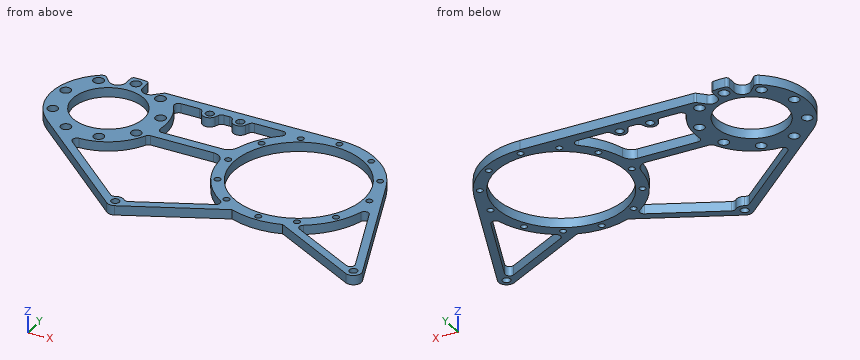
```python
from build123d import *
from build123d.topology import SkipClean

# Parameters (mm, degrees)
SKETCH2_R               = 28.575
SKETCH2_R_2             = 3.2639
SKETCH2_R_3             = 52.3875
BOSS_EXTRUDE1_DEPTH     = 7.62
CUT_EXTRUDE1_DEPTH      = 369.573342704
CUT_EXTRUDE1_DEPTH_BACK = 369.573342704
SKETCH3_R               = 4.15
SKETCH3_R_2             = 2.5
CUT_EXTRUDE2_DEPTH      = 369.573342704
CUT_EXTRUDE2_DEPTH_BACK = 369.573342704
BOSS_EXTRUDE2_DEPTH     = 7.62
CUT_EXTRUDE3_DEPTH      = 369.573342704
CUT_EXTRUDE3_DEPTH_BACK = 369.573342704
SKETCH12_R              = 3.2639


with BuildPart() as part:
    # Sketch2 → Boss-Extrude1 (new body)
    with BuildSketch(Plane.XY):
        with BuildLine():
            Line((-308.866129262, 91.710399516), (-215.926365234, 14.107506231))
            ThreePointArc((-215.926365234, 14.107506231), (-212.572921228, 12.657721799), (-208.970475069, 13.265869211))
            Line((-208.970475069, 13.265869211), (-134.814952137, 49.535152614))
            ThreePointArc((-134.814952137, 49.535152614), (-114.3, 46.0375), (-93.785047863, 49.535152614))
            Line((-93.785047863, 49.535152614), (-21.949808906, 13.301039962))
            ThreePointArc((-21.949808906, 13.301039962), (-14.699565425, 14.303090245), (-13.070560605, 21.438668609))
            Line((-13.070560605, 21.438668609), (-56.805390428, 130.917967399))
            ThreePointArc((-56.805390428, 130.917967399), (-80.468257666, 159.801430712), (-116.436314755, 169.825631839))
            Line((-116.436314755, 169.825631839), (-254.491729173, 165.059137987))
            ThreePointArc((-254.491729173, 165.059137987), (-255.416448823, 164.850182772), (-256.200136715, 164.316701751))
            Line((-256.200136715, 164.316701751), (-261.465020333, 159.051818133))
            ThreePointArc((-261.465020333, 159.051818133), (-268.548656721, 157.642795249), (-272.56121441, 163.648012211))
            Line((-272.56121441, 163.648012211), (-272.56121441, 170.220745001))
            ThreePointArc((-272.56121441, 170.220745001), (-273.218379704, 171.925600851), (-274.84982344, 172.748273949))
            ThreePointArc((-274.84982344, 172.748273949), (-279.4, 172.974), (-283.95017656, 172.748273949))
            ThreePointArc((-283.95017656, 172.748273949), (-285.581620296, 171.925600851), (-286.23878559, 170.220745001))
            Line((-286.23878559, 170.220745001), (-286.23878559, 163.648012211))
            ThreePointArc((-286.23878559, 163.648012211), (-290.251343279, 157.642795249), (-297.334979667, 159.051818133))
            Line((-297.334979667, 159.051818133), (-302.027964646, 163.744803112))
            ThreePointArc((-302.027964646, 163.744803112), (-304.229986022, 164.757469568), (-306.560860086, 164.09307692))
            ThreePointArc((-306.560860086, 164.09307692), (-325.350701602, 128.463454238), (-308.866129262, 91.710399516))
        make_face()
        with Locations(Location((-279.4, 127, 0), (0, 0, 180))):
            Circle(SKETCH2_R, mode=Mode.SUBTRACT)
        with Locations(Location((-19.05, 19.05, 0), (0, 0, 180))):
            Circle(SKETCH2_R_2, mode=Mode.SUBTRACT)
        with Locations(Location((-211.799479175, 19.05, 0), (0, 0, 180))):
            Circle(SKETCH2_R_2, mode=Mode.SUBTRACT)
        with Locations(Location((-114.3, 107.95, 0), (0, 0, 180))):
            Circle(SKETCH2_R_3, mode=Mode.SUBTRACT)
    extrude(amount=BOSS_EXTRUDE1_DEPTH)

    # Sketch3 → Cut-Extrude1 (cut, two sides: drawn at the far end of the back side and taken through both)
    with BuildSketch(Plane.XY.offset(7.62).offset(-CUT_EXTRUDE1_DEPTH_BACK)):
        with Locations((-279.4, 166)):
            Circle(SKETCH3_R)
        with Locations((-254.331283222, 156.875733282)):
            Circle(SKETCH3_R)
        with Locations((-240.992497633, 133.772278929)):
            Circle(SKETCH3_R)
        with Locations((-245.625009252, 107.5)):
            Circle(SKETCH3_R)
        with Locations((-266.06121441, 90.351987789)):
            Circle(SKETCH3_R)
        with Locations((-292.73878559, 90.351987789)):
            Circle(SKETCH3_R)
        with Locations((-313.174990748, 107.5)):
            Circle(SKETCH3_R)
        with Locations((-317.807502367, 133.772278929)):
            Circle(SKETCH3_R)
        with Locations((-304.468716778, 156.875733282)):
            Circle(SKETCH3_R)
        with Locations((-114.3, 165.1)):
            Circle(SKETCH3_R_2)
        with Locations((-57.15, 107.95)):
            Circle(SKETCH3_R_2)
        with Locations((-114.3, 50.8)):
            Circle(SKETCH3_R_2)
        with Locations((-171.45, 107.95)):
            Circle(SKETCH3_R_2)
        with Locations((-83.173879149, 155.880022958)):
            Circle(SKETCH3_R_2)
        with Locations((-64.075602011, 135.219623149)):
            Circle(SKETCH3_R_2)
        with Locations((-66.369977042, 76.823879149)):
            Circle(SKETCH3_R_2)
        with Locations((-87.030376851, 57.725602011)):
            Circle(SKETCH3_R_2)
        with Locations((-145.426120851, 60.019977042)):
            Circle(SKETCH3_R_2)
        with Locations((-164.524397989, 80.680376851)):
            Circle(SKETCH3_R_2)
        with Locations((-162.230022958, 139.076120851)):
            Circle(SKETCH3_R_2)
        with Locations((-141.569623149, 158.174397989)):
            Circle(SKETCH3_R_2)
    extrude(amount=CUT_EXTRUDE1_DEPTH + CUT_EXTRUDE1_DEPTH_BACK, mode=Mode.SUBTRACT)

    # Sketch4 → Cut-Extrude2 (cut, two sides: drawn at the far end of the back side and taken through both)
    with BuildSketch(Plane.XY.offset(7.62).offset(-CUT_EXTRUDE2_DEPTH_BACK)):
        with BuildLine():
            Line((-278.862624236, 74.930604639), (-219.018129111, 24.961616472))
            ThreePointArc((-219.018129111, 24.961616472), (-217.07692299, 24.16262829), (-215.028330647, 24.620812453))
            ThreePointArc((-215.028330647, 24.620812453), (-211.026037121, 25.442278201), (-207.335161059, 23.689967346))
            ThreePointArc((-207.335161059, 23.689967346), (-205.454963796, 22.756414152), (-203.379217054, 23.069365873))
            Line((-203.379217054, 23.069365873), (-148.393096208, 49.962941986))
            ThreePointArc((-148.393096208, 49.962941986), (-146.441473652, 52.888826728), (-148.025123052, 56.029158988))
            ThreePointArc((-148.025123052, 56.029158988), (-167.425190554, 76.155790074), (-175.994929719, 102.764124644))
            ThreePointArc((-175.994929719, 102.764124644), (-178.950352695, 108.666494642), (-185.160441746, 110.904192242))
            Line((-185.160441746, 110.904192242), (-234.876032851, 109.187714403))
            ThreePointArc((-234.876032851, 109.187714403), (-236.669637565, 108.61854745), (-237.907571885, 107.201336279))
            ThreePointArc((-237.907571885, 107.201336279), (-253.78883961, 88.82046177), (-276.820157686, 81.098441316))
            ThreePointArc((-276.820157686, 81.098441316), (-279.939618833, 78.709346862), (-278.862624236, 74.930604639))
        make_face()
        with BuildLine():
            Line((-48.019318761, 91.807143198), (-22.303873454, 27.434904147))
            ThreePointArc((-22.303873454, 27.434904147), (-23.187455951, 23.564521405), (-27.120033775, 23.021003007))
            Line((-27.120033775, 23.021003007), (-80.387932313, 49.889641079))
            ThreePointArc((-80.387932313, 49.889641079), (-82.302626367, 52.822384958), (-80.709884678, 55.941714036))
            ThreePointArc((-80.709884678, 55.941714036), (-64.405072396, 71.294115674), (-54.62867895, 91.442695545))
            ThreePointArc((-54.62867895, 91.442695545), (-51.454892751, 93.998716793), (-48.019318761, 91.807143198))
        make_face()
        with BuildLine():
            Line((-238.402359266, 157.990098388), (-157.34562354, 160.788658909))
            ThreePointArc((-157.34562354, 160.788658909), (-153.975579676, 158.578116117), (-154.932995767, 154.663138529))
            ThreePointArc((-154.932995767, 154.663138529), (-166.508163426, 141.228601653), (-173.800186524, 125.063896689))
            ThreePointArc((-173.800186524, 125.063896689), (-176.874809559, 120.512552862), (-182.037050163, 118.636570616))
            Line((-182.037050163, 118.636570616), (-230.24689137, 116.972080217))
            ThreePointArc((-230.24689137, 116.972080217), (-232.955010122, 118.116900866), (-233.829266544, 120.924069761))
            ThreePointArc((-233.829266544, 120.924069761), (-234.620613955, 137.412264953), (-241.184927886, 152.558109071))
            ThreePointArc((-241.184927886, 152.558109071), (-241.390248986, 156.091974283), (-238.402359266, 157.990098388))
        make_face()
    extrude(amount=CUT_EXTRUDE2_DEPTH + CUT_EXTRUDE2_DEPTH_BACK, mode=Mode.SUBTRACT)

    # Sketch11 → Boss-Extrude2 (add)
    with BuildSketch(Plane(origin=(0, 0, 0), x_dir=(-1, 0, 0), z_dir=(0, 0, -1))):
        with BuildLine():
            Line((207.527120949, 156.980199935), (208.688714257, 154.101435278))
            ThreePointArc((208.688714257, 154.101435278), (213.870721133, 150.472754139), (219.290640683, 153.735420862))
            Line((219.290640683, 153.735420862), (220.647990696, 156.527200807))
            ThreePointArc((220.647990696, 156.527200807), (221.987721601, 157.992282798), (223.909468964, 158.49051087))
            Line((223.909468964, 158.49051087), (221.735746538, 158.565579296))
            Line((221.735746538, 158.565579296), (216.188353984, 158.757094079))
            ThreePointArc((216.188353984, 158.757094079), (213.958358328, 153.011241823), (212.129932329, 158.897204543))
            Line((212.129932329, 158.897204543), (206.582539776, 159.088719327))
            Line((206.582539776, 159.088719327), (204.408842654, 159.163760977))
            ThreePointArc((204.408842654, 159.163760977), (206.291633306, 158.534177501), (207.527120949, 156.980199935))
        make_face()
        with BuildLine():
            ThreePointArc((199.725649115, 159.325448413), (197.803922582, 158.827213892), (196.464204543, 157.362145264))
            Line((196.464204543, 157.362145264), (195.106835972, 154.570345104))
            ThreePointArc((195.106835972, 154.570345104), (189.686908084, 151.307692234), (184.504910482, 154.936386616))
            Line((184.504910482, 154.936386616), (183.343323694, 157.815156094))
            ThreePointArc((183.343323694, 157.815156094), (182.107841163, 159.369135959), (180.225053803, 159.998724924))
            Line((180.225053803, 159.998724924), (182.398748746, 159.923676049))
            Line((182.398748746, 159.923676049), (187.94614081, 159.732147087))
            ThreePointArc((187.94614081, 159.732147087), (189.774551766, 153.846179694), (192.004562108, 159.59202625))
            Line((192.004562108, 159.59202625), (197.551954171, 159.400497289))
            Line((197.551954171, 159.400497289), (199.725649115, 159.325448413))
        make_face()
    extrude(amount=-BOSS_EXTRUDE2_DEPTH)

    # Sketch12 → Cut-Extrude3 (cut, two sides: drawn at the far end of the back side and taken through both)
    with SkipClean():  # the faces are left unmerged after this step: merging them gives an invalid solid
        with BuildSketch(Plane(origin=(0, 0, 0), x_dir=(-1, 0, 0), z_dir=(0, 0, -1)).offset(-CUT_EXTRUDE3_DEPTH_BACK)):
            with Locations((189.887173898, 157.10813608)):
                Circle(SKETCH12_R)
            with Locations((214.070972123, 156.273198497)):
                Circle(SKETCH12_R)
        extrude(amount=CUT_EXTRUDE3_DEPTH + CUT_EXTRUDE3_DEPTH_BACK, mode=Mode.SUBTRACT)


solid = part.part
```
Geometry check sheet. Reference: the model listing, model coordinates, mm. Give positions to 0.01 mm unless a question says otherwise; leave off trailing zeros. Loops run counter-clockwise (first coordinate to the right, second up) from the corner with the lowest first, then second, coordinate; pieces in that order, holes last. Notation, with made-up numbers: (0.5, -32) - (21.5, -32) arc R16 cw to (21.5, -10) - close; hole circle Ø8 at (84.5, 26.5). An arc over 180 degrees is marked (long way). Use CSV: the item, a comma, the result in double quotes. Start each with the question number.
Q1. Scan lines: probe 1 along Y at (x, z) = (-114.5, 4.5); probe 2 along Y at (x, z) = (-229, 6.75); probe 3 along Y at (x, z) = (-84, 0.5). Record each from-to range of solid material in increasing order. Write a range as from..to.
Q2. Section check B-B, the plane z = 2. Count the separate pieces of the cut face and the enclosed holes in it, and give its area (3 significant figures).
Q3. Go/stop test with flat-tipped pins: pin 1 Ø1 at (x, z) = (-166, 6.5) entering from +Y; pin 2 Ø4 at (x, z) = (-236, 6) entering from +Y; pin 3 Ø1.5 at (y, z) = (103.5, 3.5) entering from -X. Record where each tip stops, or that it passes through.
Q4. Section check A-A, the plane x = -34.5. Record the cut outline in (y, z).
Findings below:
1,probe 1,"y = 46.04..48.31, 53.29..55.56, 160.34..162.61, 167.59..169.86"
1,probe 2,"y = 25.02..33.3, 109.39..117.02, 158.31..165.94"
1,probe 3,"y = 44.6..65.21, 150.69..153.52, 158.24..161.94"
2,separate pieces,"1"
2,enclosed holes,"30"
2,area,"10,300 mm^2"
3,pin 1,"stops at y = 168.13"
3,pin 2,"stops at y = 165.77"
3,pin 3,"stops at x = -319.35"
4,outline,"(19.63, 0) - (26.74, 0) - (26.74, 7.62) - (19.63, 7.62) - close; (57.96, 0) - (75.08, 0) - (75.08, 7.62) - (57.96, 7.62) - close"
